For this review, take the finished solid that the model builds, in its own axes (mm). Give positions to 0.01 mm unless a question says otherwise; leave off trailing zeros. Loops run counter-clockwise (first coordinate to the right, second up) from the corner with the lowest first, then second, coordinate; pieces in that order, holes last. Notation, with made-up numbers: (19, 71) - (44, 71) arc R7 ccw to (44, 80) - close; hole circle Ø4 at (-25.75, -7.5). An arc over 180 degrees is marked (long way). Use CSV: the item, a comma, the result in double quotes. Start each with the question number.
1. For pin 1 (3 mm diameter, centred on x = -9.5, z = -17.5, fed in from +Y); pin 2 (6 mm diameter, centred on x = 52.5, y = -4, fed in from -Z); pin 3 (3 mm diameter, centred on y = -14, z = -6, fed in from +X); pin 4 (5 mm diameter, centred on x = -7.5, y = -16.5, fed in from -Z), all flat-tipped, find the tip position at first contact; note any pin that passes through.
2. Mouldability with a two-part tool opening along X and no side actions: class faces 1 (the cylindrical face through (46.37, -12.68, -2)), 2 (the flat face through (40, 0, 6)), 3 (the flat face through (46.15, -12.32, -21.23)) as pulls with the +X half, pulls with the -X half, needs draft (parallel to the pull), parting line crosses it, or undercut.
3. Take a section at B-B on y = -16.75. Give the boundary of the cut face in (x, z), plus the area to 3 significant figures.
4. Wall thickness on line 1 (X direction, y = -7.5, z = 1); line 2 (Z direction, x = 90, y = -5.75); line 3 (Z direction, x = -5.5, y = -3.25): over which ranges is each line inside the solid? List them lowest first.
5. Take a section at C-C on z = -8. State how many separate pieces and enclosed holes the cut face has, plus the area to 3 significant figures.
6. Take a section at D-D on x = 90. Give the boundary of the cut face in (y, z).
7. Take a section at A-A on x = 0. Give the boundary of the cut face in (y, z).
```python
from build123d import *

# Parameters (mm, degrees)
F0_R     = 10
F1_DEPTH = 25
F2_SIZE  = 2
F6_R     = 5.2276340185
F7_DEPTH = 25


# Not quite as in the source:
# - the program builds the solid bodies; features that only make, move or delete a surface that nothing else refers to are left out


with BuildPart() as f1:
    # F0 (on Front) → F1 (new body)
    with BuildSketch(Plane.XZ):
        with BuildLine():
            ThreePointArc((2.0833333333, -24.9130432148), (18.3995018048, -16.9250800097), (25, 0))
            ThreePointArc((25, 0), (18.3995018048, 16.9250800097), (2.0833333333, 24.9130432148))
            ThreePointArc((2.0833333333, 24.9130432148), (-25, 0), (2.0833333333, -24.9130432148))
        make_face()
        Circle(F0_R, mode=Mode.SUBTRACT)
        with BuildLine():
            ThreePointArc((2.0833333333, 24.9130432148), (18.3995018048, 16.9250800097), (25, 0))
            ThreePointArc((25, 0), (18.3995018048, -16.9250800097), (2.0833333333, -24.9130432148))
            Line((2.0833333333, -24.9130432148), (91.4583333333, -17.4391302504))
            ThreePointArc((91.4583333333, -17.4391302504), (72.5, 0), (91.4583333333, 17.4391302504))
            Line((91.4583333333, 17.4391302504), (2.0833333333, 24.9130432148))
        make_face()
        with BuildLine():
            ThreePointArc((107.5, 0), (102.8796512634, 11.8475560068), (91.4583333333, 17.4391302504))
            ThreePointArc((91.4583333333, 17.4391302504), (72.5, 0), (91.4583333333, -17.4391302504))
            ThreePointArc((91.4583333333, -17.4391302504), (102.8796512634, -11.8475560068), (107.5, 0))
        make_face()
        with Locations((90, 0)):
            Circle(F0_R, mode=Mode.SUBTRACT)
    extrude(amount=F1_DEPTH)

    # F2
    f2_edges = [f1.edges().sort_by_distance(p)[0] for p in [
        (80, -25, 0),
    ]]
    chamfer(f2_edges, length=F2_SIZE)

    # F6 (on face) → F7 (cut)
    with BuildSketch(Plane.XZ.offset(25)):
        with Locations((41.5417253971, 0)):
            Circle(F6_R)
    extrude(amount=-F7_DEPTH, mode=Mode.SUBTRACT)


solid = f1.part
```
Check result:
1,pin 1,"stops at y = 0"
1,pin 2,"stops at z = -20.95"
1,pin 3,"stops at x = 106.91"
1,pin 4,"stops at z = -24.49"
2,face 1,"undercut"
2,face 2,"needs draft"
2,face 3,"pulls with the +X half"
3,outline,"(2.08, -24.91) - (91.46, -17.44) arc R17.5 ccw to (91.46, 17.44) - (2.08, 24.91) arc R25 ccw (long way) to start; hole circle Ø20 at (0, 0); hole circle Ø10.46 at (41.54, 0); hole circle Ø20 at (90, 0)"
3,area,"4,590 mm²"
4,line 1,"x = -24.98 to -9.95, 9.95 to 36.41, 46.67 to 80.05, 99.95 to 107.47"
4,line 2,"z = -17.56 to -10, 10 to 17.56"
4,line 3,"z = -24.39 to -8.35, 8.35 to 24.39"
5,separate pieces,"3"
5,enclosed holes,"0"
5,area,"2,630 mm²"
6,outline,"(-25, -17.56) - (0, -17.56) - (0, -10) - (-23, -10) - (-25, -12) - close; (-25, 12) - (-23, 10) - (0, 10) - (0, 17.56) - (-25, 17.56) - close"
7,outline,"(-25, -25) - (0, -25) - (0, -10) - (-25, -10) - close; (-25, 10) - (0, 10) - (0, 25) - (-25, 25) - close"
